Check sheet for the modelled part. Datum: model origin and axes. Units: mm. A direction names the side the tool comes from. Coordinates: 2 decimals unless noted, no trailing zeros. Write each loop counter-clockwise with the first axis right and the second up, starting at its lowest first coordinate (ties: lowest second). Pieces come first, ordered by that corner, then holes. Notation, with made-up numbers: M 37.5,-6 L 54.5,-6 A20 ccw 54.5,-2 Z; hole C 80.5,40.25 d3. An arc over 180 degrees is marked long. Answer as CSV lines item,"result".
Autodesk Inventor part; units mm, degrees
ref_plane "Start Plane" through (0, 0, 153.3871) normal (0, 0, 1) x (1, 0, 0)
ref_plane "End Plane" through (0, 0, 2520) normal (0, 0, 1) x (1, 0, 0)
ref_plane "Work Plane4" through (25.5143, 34, 159.3429) normal (0.0905, 0, -0.9959) x (-0.9959, 0, -0.0905)
ref_plane "Start Plane" through (0, 0, 153.3871) normal (0, 0, 1) x (1, 0, 0)
ref_plane "End Plane" through (0, 0, 2520) normal (0, 0, 1) x (1, 0, 0)
sketch "Sketch" plane through (0, 0, 0) normal (0, 0, 1) x (1, 0, 0)
  line L0 (-40, -34) -> (-40, 34)
  line L1 (-34, 40) -> (34, 40)
  line L2 (40, 34) -> (40, -34)
  line L3 (34, -40) -> (-34, -40)
  arc A0 (-40, -34) -> (-34, -40) centre (-34, -34) ccw
  arc A1 (40, 34) -> (34, 40) centre (34, 34) ccw
  arc A2 (-34, 40) -> (-40, 34) centre (-34, 34) ccw
  arc A3 (34, -40) -> (40, -34) centre (34, -34) ccw
  arc A4 (-34, 37) -> (-37, 34) centre (-34, 34) ccw
  line L4 (-34, 37) -> (34, 37)
  arc A5 (37, 34) -> (34, 37) centre (34, 34) ccw
  line L5 (37, 34) -> (37, -34)
  arc A6 (34, -37) -> (37, -34) centre (34, -34) ccw
  line L6 (34, -37) -> (-34, -37)
  arc A7 (-37, -34) -> (-34, -37) centre (-34, -34) ccw
  line L7 (-37, -34) -> (-37, 34)
  line L8 (0, 57.7397) -> (0, -57.7397) construction
  line L9 (-57.7397, 0) -> (57.7397, 0) construction
  dimension "d7" = 6
  dimension "d9" = 80
  dimension "d11" = 80
  dimension "d12" = 3
  dimension "d15" = 40
  dimension "d16" = 40
extrude "Body" add sketch "Sketch" along normal up to surface (2366.6129 mm away) from surface at 153.3871
sketch "Sketch3" plane through (0, 0, 0) normal (0, 0, 1) x (1, 0, 0)
  line L0 (0, 0) -> (10, 0)
ref_plane "Work Plane3" through (0, 0, 0) normal (0, -1, 0) x (1, 0, 0)
ref_plane "Work Plane4" through (25.5143, 34, 159.3429) normal (0.0905, 0, -0.9959) x (-0.9959, 0, -0.0905)
split "Split1" plane through (25.5143, 34, 159.3429) removes the side toward (0.0905, 0, -0.9959)
ref_plane "Work Plane5" through (-2160, 34, 2520) normal (0, 0, 1) x (1, 0, 0)
split "Split2" plane through (-2160, 34, 2520) removes the side toward (0, 0, 1)
sketch "Sketch4" plane through (0, 0, 0) normal (0, -1, 0) x (1, 0, 0)
  line L0 (-2, 153.3871) -> (12, 153.3871)
  line L1 (-2, 2520) -> (12, 2520)
  dimension "d18" = 2366.6129
equation "\"d7\" = G_IR"
equation "\"d9\" = G_W"
equation "\"d11\" = G_H"
equation "\"d12\" = G_T"
equation "\"d15\" = 0.5 * d9"
equation "\"d16\" = 0.5 * d11"
equation "\"d3\" = G_L"
equation "\"G_W\" = 80"
equation "\"G_H\" = 80"
equation "\"G_T\" = 3"
equation "\"G_IR\" = 6"
equation "\"G_L\" = d18"
equation "\"G_OFFSET_START\" = -153.38707"
equation "\"d13\" = -G_OFFSET_START"
properties part number "ISO 10799-2 - 80x80x3 - 2366,61" material "Steel, Mild"
1) Section check B-B, the plane z = 1742. Record the boundary of the cut face in (x, y), plus the area to 3 significant figures.
Answer key:
outline,"M -40,-34 A6 ccw -34,-40 L 34,-40 A6 ccw 40,-34 L 40,34 A6 ccw 34,40 L -34,40 A6 ccw -40,34 Z; hole M -37,-34 A3 ccw -34,-37 L 34,-37 A3 ccw 37,-34 L 37,34 A3 ccw 34,37 L -34,37 A3 ccw -37,34 Z"
area,"901 mm2"
2) Thickness scan on line 1 along Y through (x, z) = (-31, 1946.5); line 2 along X through (y, z) = (-35, 1797). Record the ranges inside material, lowest first.
Answer key:
line 1,"y = -40 to -37, 37 to 40"
line 2,"x = -39.92 to -36.83, 36.83 to 39.92"
3) Tool access check on faces 1 (the face through (-37, 0, 1320)), 2 (the face through (-38.705, 0.187, 153.507)). Record the directions out of +Z, -Z, +X, -X, +Y, -Y that give a thin tool (end or side, any length) a straight path to the whole face; none if there is none.
Answer key:
face 1,"+Z, -Z"
face 2,"-Z, +X, +Y, -Y"
4) Section check A-A, the plane y = -15.5. Record the boundary of the cut face in (x, z), plus the area to 3 significant figures.
Answer key:
outline,"M -40,153.39 L -37,153.66 L -37,2520 L -40,2520 Z; M 37,160.39 L 40,160.66 L 40,2520 L 37,2520 Z"
area,"14,200 mm2"
5) Section check C-C, the plane x = -17. Record the boundary of the cut face in (y, z), plus the area to 3 significant figures.
Answer key:
outline,"M -40,155.48 L -37,155.48 L -37,2520 L -40,2520 Z; M 37,155.48 L 40,155.48 L 40,2520 L 37,2520 Z"
area,"14,200 mm2"
6) Mould release check, pull along Y, two halves, no side actions. Record for faces 3 (the face through (0, 40, 1320)), 4 (the face through (40, 0, 1324)), 5 (the face through (0, -37, 1320)): pulls with the +Y half, pulls with the -Y half, needs draft (parallel to the pull), parting line crosses it, or undercut.
Answer key:
face 3,"pulls with the +Y half"
face 4,"needs draft"
face 5,"undercut"
7) Depth check by flat-ended pin: P1, Ø8, axis at x = 9, y = 30.5, coming from the -Z side. Enter the tip coordinate at first touch or a pass-through.
Answer key:
P1,"passes through"
